The model under review builds one solid part; all positions refer to its coordinate system, in mm. A direction names the side the tool comes from. Round coordinates to 2 decimals unless told otherwise and drop trailing zeros. Write each loop counter-clockwise with the first axis right and the second up, starting at its lowest first coordinate (ties: lowest second). Pieces come first, ordered by that corner, then holes. Notation, with made-up numbers: (24.25, -34) - (58.25, -34) arc R26 ccw to (58.25, -11) - close; hole circle Ø8 at (48, 74.25). An arc over 180 degrees is marked (long way). Return JSON: item names as keys, results as strings.
from build123d import *

# Parameters (mm, degrees)
SKETCH1_W                    = 50.8
SKETCH1_H                    = 25.4
SKETCH1_W_2                  = 44.45
SKETCH1_H_2                  = 19.05
BOSS_EXTRUDE1_DEPTH          = 697.2046
CUT_EXTRUDE1_DEPTH           = 699.129339207
CUT_EXTRUDE3_DEPTH           = 699.129339207
F_10_0_1935_DIAMETER_HOLE1_D = 4.9149


with BuildPart() as part:
    # Sketch1 → Boss-Extrude1 (new body)
    with BuildSketch(Plane.XY):
        Rectangle(SKETCH1_W, SKETCH1_H)
        Rectangle(SKETCH1_W_2, SKETCH1_H_2, mode=Mode.SUBTRACT)
    extrude(amount=BOSS_EXTRUDE1_DEPTH)

    # Sketch2 → Cut-Extrude1 (cut, through all)
    with BuildSketch(Plane(origin=(0, 12.7, 0), x_dir=(1, 0, 0), z_dir=(0, 1, 0))):
        Polygon((-25.4, -697.2046), (25.4, -646.4046), (25.4, -697.2046), align=None)
        Polygon((25.4, 0), (-25.4, -50.8), (-25.4, 0), align=None)
    extrude(amount=-CUT_EXTRUDE1_DEPTH, mode=Mode.SUBTRACT)

    # Sketch3 → Cut-Extrude3 (cut, through all)
    with BuildSketch(Plane(origin=(0, 12.7, 0), x_dir=(1, 0, 0), z_dir=(0, 1, 0))):
        Polygon((25.4, 0), (25.4, -25.2984), (12.7508, -12.6492), align=None)
    extrude(amount=-CUT_EXTRUDE3_DEPTH, mode=Mode.SUBTRACT)

    # #10 (0.1935) Diameter Hole1 (through all)
    with Locations(Plane(origin=(0, -12.7, 0), x_dir=(-1, 0, 0), z_dir=(0, -1, 0))):
        with Locations((0, -604.320502063), (0, -636.070502063)):
            Hole(F_10_0_1935_DIAMETER_HOLE1_D / 2)


solid = part.part
(1) Add section C-C (x = -9). Write out the cut boundary in (y, z) (3 decimals).
Filled in:
{"outline": "(-12.7, 34.4) - (-9.525, 34.4) - (-9.525, 680.805) - (-12.7, 680.805) - close; (9.525, 34.4) - (12.7, 34.4) - (12.7, 680.805) - (9.525, 680.805) - close"}
(2) Add section A-A (y = -4.25). Write out the cut boundary in (x, z) (3 decimals), plus the area to 3 significant figures.
Filled in:
{"outline": "(-25.4, 50.8) - (-22.225, 47.625) - (-22.225, 694.03) - (-25.4, 697.205) - close; (22.225, 22.123) - (25.4, 25.298) - (25.4, 646.405) - (22.225, 649.58) - close", "area": "4,030 mm2"}
(3) Mouldability with a two-part tool opening along Y and no side actions: class faces 3 (the flat face through (23.4, 0.2, 23.3)), 4 (the flat face through (0, 9.525, 349)), 5 (the flat face through (0, -12.7, 350)) as released by +Y, released by -Y, zero draft, split by the parting line, or undercut.
Filled in:
{"face 3": "zero draft", "face 4": "undercut", "face 5": "released by -Y"}
(4) Clearance check with flat-ended pins moving along their axes: pin 1 Ø8 at (x, z) = (0, 604.32) entering from -Y; pin 2 Ø3 at (x, z) = (0, 636.07) entering from -Y; pin 3 Ø8 at (x, y) = (12, 8) entering from +Z. State where each tip first meets the part, or that it passes through.
Filled in:
{"pin 1": "stops at y = -12.7", "pin 2": "passes through", "pin 3": "stops at z = 663.5"}
(5) For faces 1 (the flat face through (-25.4, 0, 369)), 2 (the flat face through (0, -9.525, 349)), list the 3-axis set-ups (+Z, -Z, +X, -X, +Y, -Y) from which the entire face can be reached by the end or side of a thin tool; tool diameter is ignored.
Filled in:
{"face 1": "+Z, -Z, -X, +Y, -Y", "face 2": "+Z, -Z"}
(6) Wall thickness on line 1 (Y direction, x = -15, z = 119.5) (3 decimals); line 2 (Z direction, x = 0, y = 10.9); line 3 (X direction, y = -7, z = 453) (3 decimals): over which ranges is each line inside the solid? List them lowest first.
Filled in:
{"line 1": "y = -12.7 to -9.525, 9.525 to 12.7", "line 2": "z = 25.4 to 601.86, 606.78 to 633.61, 638.53 to 671.8", "line 3": "x = -25.4 to -22.225, 22.225 to 25.4"}
(7) Add section B-B (z = 103.5). Write out the cut boundary in (x, y) (3 decimals), plus the area to 3 significant figures.
Filled in:
{"outline": "(-25.4, -12.7) - (25.4, -12.7) - (25.4, 12.7) - (-25.4, 12.7) - close; hole (-22.225, -9.525) - (22.225, -9.525) - (22.225, 9.525) - (-22.225, 9.525) - close", "area": "444 mm2"}
